```python
from build123d import *

# Parameters (mm, degrees)
F0_R     = 10
F1_DEPTH = 25
F3_DEPTH = 10
F4_SIZE  = 7


with BuildPart() as f1:
    # F0 (on Front) → F1 (new body)
    with BuildSketch(Plane.XZ):
        Circle(F0_R)
    extrude(amount=F1_DEPTH)

    # F2 (on Front) → F3 (join)
    with BuildSketch(Plane.XZ):
        with BuildLine():
            Line((-50.8304547985, -10.7641287668), (-2.4913643956, -14.7923863004))
            ThreePointArc((-2.4913643956, -14.7923863004), (0, -14.896013553), (2.4913643956, -14.7923863004))
            Line((2.4913643956, -14.7923863004), (50.8304547985, -10.7641287668))
            ThreePointArc((50.8304547985, -10.7641287668), (57.3588228673, -7.5697660742), (60, -0.7986711843))
            Line((60, -0.7986711843), (60, 0.7986711843))
            ThreePointArc((60, 0.7986711843), (57.3588228673, 7.5697660742), (50.8304547985, 10.7641287668))
            Line((50.8304547985, 10.7641287668), (2.4913643956, 14.7923863004))
            ThreePointArc((2.4913643956, 14.7923863004), (0, 14.896013553), (-2.4913643956, 14.7923863004))
            Line((-2.4913643956, 14.7923863004), (-50.8304547985, 10.7641287668))
            ThreePointArc((-50.8304547985, 10.7641287668), (-57.3588228673, 7.5697660742), (-60, 0.7986711843))
            Line((-60, 0.7986711843), (-60, -0.7986711843))
            ThreePointArc((-60, -0.7986711843), (-57.3588228673, -7.5697660742), (-50.8304547985, -10.7641287668))
        make_face()
    extrude(amount=-F3_DEPTH)

    # F4
    f4_edges = [f1.edges().sort_by_distance(p)[0] for p in [
        (-26.66091, 10, -12.778258),
        (0, 10, -14.896014),
        (26.66091, 10, -12.778258),
        (57.358823, 10, -7.569766),
        (60, 10, 0),
        (57.358823, 10, 7.569766),
        (26.66091, 10, 12.778258),
        (0, 10, 14.896014),
        (-26.66091, 10, 12.778258),
        (-57.358823, 10, 7.569766),
        (-60, 10, 0),
        (-57.358823, 10, -7.569766),
    ]]
    chamfer(f4_edges, length=F4_SIZE)


solid = f1.part
```
For this review, take the finished solid that the model builds, in its own axes (mm). A direction names the side the tool comes from. Round coordinates to 2 decimals unless told otherwise and drop trailing zeros. Order: outer loops, then holes, each group sorted by start corner. A loop starts at its lowest first (then second) coordinate and runs counter-clockwise, first axis right, second up.
Q1. We need section B-B, the plane y = -9. Give the boundary of the cut face in (x, z), plus the area to 3 significant figures.
Findings below:
outline: circle Ø20 at (0, 0)
area: 314 mm2
Q2. Insertion check: P1, Ø8, axis at x = -15.5, z = 10, coming from the -Y side; P2, Ø3, axis at y = -6, z = 1, coming from the -X side; P3, Ø8, axis at y = -4.5, z = -1, coming from the +X side. Each pin has a flat end and moves straight along its axis. Give the tip position at first contact, or say it passes through.
Findings below:
P1: stops at y = 0
P2: stops at x = -10
P3: stops at x = 10
Q3. We need section A-A, the plane x = 0. Give the boundary of the cut face in (y, z), plus the area to 3 significant figures.
Findings below:
outline: (-25, -10) - (0, -10) - (0, -14.9) - (3, -14.9) - (10, -7.9) - (10, 7.9) - (3, 14.9) - (0, 14.9) - (0, 10) - (-25, 10) - close
area: 749 mm2
Q4. Machinability: for faces 1 (the cylindrical face through (-2.17, -12.32, -9.76)), 2 (the conical face through (-54.7, 6.55, 5.22)), which of the approach directions +Z, -Z, +X, -X, +Y, -Y give a long, thin tool a straight path to every point of the face, cutting with its end or side? Answer none if there is none.
Findings below:
face 1: -Y
face 2: +Z, -X, +Y
Q5. We need section C-C, the plane x = 35. Give the boundary of the cut face in (y, z).
Findings below:
outline: (0, -12.08) - (3, -12.08) - (10, -5.06) - (10, 5.06) - (3, 12.08) - (0, 12.08) - close
Q6. Wall thickness on line 1 (X direction, y = -9.5, z = -6.25); line 2 (Y direction, x = -27, z = -5.75); line 3 (Z direction, x = -2.5, y = 7): over which ranges is each line inside the solid? List them lowest first.
Findings below:
line 1: x = -7.81 to 7.81
line 2: y = 0 to 9.98
line 3: z = -10.78 to 10.78
